For this review, take the finished solid that the model builds, in its own axes (mm). Coordinates: 2 decimals unless noted, no trailing zeros. Order: outer loops, then holes, each group sorted by start corner. A loop starts at its lowest first (then second) coordinate and runs counter-clockwise, first axis right, second up. Notation, with made-up numbers: (-11.75, -15.5) -> (7.25, -15.5) arc R19 cw to (7.25, 21.5) -> close; hole circle Ø1 at (-14, 79.25). An arc over 180 degrees is marked (long way). Write item = value, one per line. Start each with the question number.
1) Consider section C-C on x = 0. Give the boundary of the cut face in (y, z) (3 decimals), and give its area (3 significant figures).
2) Wall thickness on probe 1 along X at (y, z) = (-13, 4.35); probe 2 along Y at (x, z) = (0, 2.2) (3 decimals); probe 3 along X at (y, z) = (15, 2.55): over which ranges is each line inside the solid? List them lowest first. Write a range as [from, to].
3) Consider section D-D on y = -12. Give the boundary of the cut face in (x, z) (3 decimals).
4) Insertion check: pin 1 Ø11.5 at (x, y) = (30, 15) entering from +Z; pin 2 Ø8 at (x, y) = (-30, 15) entering from -Z; pin 3 Ø0.6 at (x, z) = (-36, 2.5) entering from -Y; pin 4 Ø1.7 at (x, z) = (35.5, 3.5) entering from +Y. Each pin has a flat end and moves straight along its axis. Give the tip position at first contact, or say it passes through.
5) Consider section A-A on y = -30. Give the boundary of the cut face in (x, z) (3 decimals), and give its area (3 significant figures).
6) Consider section B-B on z = 1.8. Give the boundary of the cut face in (x, y) (3 decimals), and give its area (3 significant figures).
from build123d import *

# Parameters (mm, degrees)
CROQUIS1_R              = 4.95
CROQUIS1_R_2            = 3.175
SALIENTE_EXTRUIR1_DEPTH = 5
CORTAR_EXTRUIR1_DEPTH   = 78.590270009


with BuildPart() as part:
    # Croquis1 → Saliente-Extruir1 (new body)
    with BuildSketch(Plane.XY):
        with BuildLine():
            Line((13, 0), (-13, 0))
            ThreePointArc((-13, 0), (-19.544656296, 4.709966775), (-24.061489507, 11.389377737))
            ThreePointArc((-24.061489507, 11.389377737), (-30, 21.95), (-35.938510493, 11.389377737))
            ThreePointArc((-35.938510493, 11.389377737), (-36.984260452, 5.34343649), (-40, 0))
            Line((-40, 0), (-55, 0))
            Line((-55, 0), (-55, -24))
            Line((-55, -24), (-25, -24))
            Line((-25, -24), (-25, -54.5))
            Line((-25, -54.5), (25, -54.5))
            Line((25, -54.5), (25, -24))
            Line((25, -24), (55, -24))
            Line((55, -24), (55, 0))
            Line((55, 0), (40, 0))
            ThreePointArc((40, 0), (36.984260452, 5.34343649), (35.938510493, 11.389377737))
            ThreePointArc((35.938510493, 11.389377737), (30, 21.95), (24.061489507, 11.389377737))
            ThreePointArc((24.061489507, 11.389377737), (19.544656296, 4.709966775), (13, 0))
        make_face()
        with Locations((-30, 15)):
            Circle(CROQUIS1_R, mode=Mode.SUBTRACT)
        with Locations((-37.5, -12)):
            Circle(CROQUIS1_R_2, mode=Mode.SUBTRACT)
        with Locations((0, -30)):
            Circle(CROQUIS1_R_2, mode=Mode.SUBTRACT)
        with Locations(Location((30, 15, 0), (0, 0, 180))):
            Circle(CROQUIS1_R, mode=Mode.SUBTRACT)
        with Locations(Location((37.5, -12, 0), (0, 0, 180))):
            Circle(CROQUIS1_R_2, mode=Mode.SUBTRACT)
    extrude(amount=SALIENTE_EXTRUIR1_DEPTH)

    # Croquis2 → Cortar-Extruir1 (cut, through all)
    with BuildSketch(Plane.XY):
        with BuildLine():
            Line((-30, 16.7), (-36.738879729, 16.7))
            ThreePointArc((-36.738879729, 16.7), (-36.95, 15), (-36.738879729, 13.3))
            Line((-36.738879729, 13.3), (-30, 13.3))
            Line((-30, 13.3), (-30, 16.7))
        make_face()
        with BuildLine():
            Line((30, 16.7), (30, 13.3))
            Line((30, 13.3), (36.738879729, 13.3))
            ThreePointArc((36.738879729, 13.3), (36.95, 15), (36.738879729, 16.7))
            Line((36.738879729, 16.7), (30, 16.7))
        make_face()
    extrude(amount=CORTAR_EXTRUIR1_DEPTH, mode=Mode.SUBTRACT)


solid = part.part
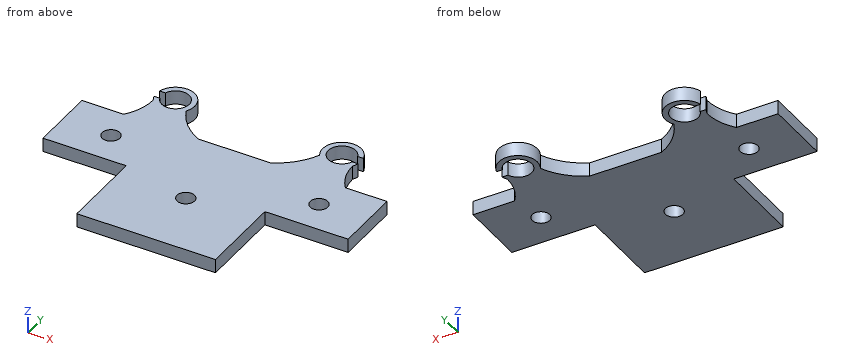
Answer sheet:
q1.outline = (-54.5, 0) -> (-33.175, 0) -> (-33.175, 5) -> (-54.5, 5) -> close; (-26.825, 0) -> (0, 0) -> (0, 5) -> (-26.825, 5) -> close
q1.area = 241 mm2
q2.probe_1 = [-55, -40.51], [-34.49, 34.49], [40.51, 55]
q2.probe_2 = [-54.5, -33.175], [-26.825, 0]
q2.probe_3 = [-25.05, -23.05], [23.05, 25.05]
q3.outline = (-55, 0) -> (-40.675, 0) -> (-40.675, 5) -> (-55, 5) -> close; (-34.325, 0) -> (34.325, 0) -> (34.325, 5) -> (-34.325, 5) -> close; (40.675, 0) -> (55, 0) -> (55, 5) -> (40.675, 5) -> close
q4.pin_1 = 5
q4.pin_2 = through
q4.pin_3 = -24
q4.pin_4 = 20.17
q5.outline = (-25, 0) -> (-3.175, 0) -> (-3.175, 5) -> (-25, 5) -> close; (3.175, 0) -> (25, 0) -> (25, 5) -> (3.175, 5) -> close
q5.area = 218 mm2
q6.outline = (-55, -24) -> (-25, -24) -> (-25, -54.5) -> (25, -54.5) -> (25, -24) -> (55, -24) -> (55, 0) -> (40, 0) arc R18 cw to (35.939, 11.389) arc R6.95 ccw to (36.739, 13.3) -> (34.649, 13.3) arc R4.95 cw (long way) to (34.649, 16.7) -> (36.739, 16.7) arc R6.95 ccw (long way) to (24.061, 11.389) arc R23 cw to (13, 0) -> (-13, 0) arc R23 cw to (-24.061, 11.389) arc R6.95 ccw (long way) to (-36.739, 16.7) -> (-34.649, 16.7) arc R4.95 cw (long way) to (-34.649, 13.3) -> (-36.739, 13.3) arc R6.95 ccw to (-35.939, 11.389) arc R18 cw to (-40, 0) -> (-55, 0) -> close; hole circle Ø6.35 at (-37.5, -12); hole circle Ø6.35 at (0, -30); hole circle Ø6.35 at (37.5, -12)
q6.area = 4,550 mm2
